from build123d import *

# Parameters (mm, degrees)
F0_W     = 10
F0_H     = 15
F1_DEPTH = 5
F2_DEPTH = 3
F4_DEPTH = 3
F5_DEPTH = 25


with BuildPart() as f1:
    # F0 (on Top) → F1 (new body)
    with BuildSketch(Plane.XY):
        Rectangle(F0_W, F0_H)
    extrude(amount=-F1_DEPTH)

    # F0 (on Top) → F2 (join)
    with BuildSketch(Plane.XY):
        with BuildLine():
            Line((-30, -50), (30, -50))
            Line((30, -50), (30, 50))
            Line((30, 50), (15, 50))
            Line((15, 50), (15, 46.55))
            ThreePointArc((15, 46.55), (16.0960155108, 46.0960155108), (16.55, 45))
            ThreePointArc((16.55, 45), (16.2263348543, 44.0520533638), (15.3905124838, 43.5))
            Line((15.3905124838, 43.5), (20.76, 43.5))
            Line((20.76, 43.5), (23.935, 43.5))
            Line((23.935, 43.5), (27.5, 43.5))
            Line((27.5, 43.5), (27.5, -43.5))
            Line((27.5, -43.5), (-27.5, -43.5))
            Line((-27.5, -43.5), (-27.5, -37.145))
            Line((-27.5, -37.145), (-27.5, 28.895))
            Line((-27.5, 28.895), (-27.5, 43.5))
            Line((-27.5, 43.5), (-24.325, 43.5))
            Line((-24.325, 43.5), (-21.15, 43.5))
            Line((-21.15, 43.5), (-15.3905124838, 43.5))
            ThreePointArc((-15.3905124838, 43.5), (-16.2263348543, 44.0520533638), (-16.55, 45))
            Line((-16.55, 45), (-30, 45))
            Line((-30, 45), (-30, -50))
        make_face()
        with BuildLine():
            Line((-30, 50), (-30, 45))
            Line((-30, 45), (-16.55, 45))
            ThreePointArc((-16.55, 45), (-16.0960155108, 46.0960155108), (-15, 46.55))
            Line((-15, 46.55), (-15, 50))
            Line((-15, 50), (-30, 50))
        make_face()
        with BuildLine():
            Line((15, 46.55), (15, 50))
            Line((15, 50), (-15, 50))
            Line((-15, 50), (-15, 46.55))
            ThreePointArc((-15, 46.55), (-13.9039844892, 46.0960155108), (-13.45, 45))
            Line((-13.45, 45), (13.45, 45))
            ThreePointArc((13.45, 45), (13.9039844892, 46.0960155108), (15, 46.55))
        make_face()
        with BuildLine():
            ThreePointArc((-14.6094875162, 43.5), (-15, 43.45), (-15.3905124838, 43.5))
            Line((-15.3905124838, 43.5), (-21.15, 43.5))
            Line((-21.15, 43.5), (-21.15, 28.895))
            Line((-21.15, 28.895), (20.76, 28.895))
            Line((20.76, 28.895), (20.76, 43.5))
            Line((20.76, 43.5), (15.3905124838, 43.5))
            ThreePointArc((15.3905124838, 43.5), (15, 43.45), (14.6094875162, 43.5))
            Line((14.6094875162, 43.5), (-14.6094875162, 43.5))
        make_face()
        with BuildLine():
            ThreePointArc((14.6094875162, 43.5), (13.7736651457, 44.0520533638), (13.45, 45))
            Line((13.45, 45), (-13.45, 45))
            ThreePointArc((-13.45, 45), (-13.7736651457, 44.0520533638), (-14.6094875162, 43.5))
            Line((-14.6094875162, 43.5), (14.6094875162, 43.5))
        make_face()
        with BuildLine():
            Line((-21.15, 28.895), (-21.15, 43.5))
            Line((-21.15, 43.5), (-24.325, 43.5))
            Line((-24.325, 43.5), (-24.325, 30.445))
            ThreePointArc((-24.325, 30.445), (-23.2289844892, 29.9910155108), (-22.775, 28.895))
            Line((-22.775, 28.895), (-21.15, 28.895))
        make_face()
        with BuildLine():
            Line((-24.325, 30.445), (-24.325, 43.5))
            Line((-24.325, 43.5), (-27.5, 43.5))
            Line((-27.5, 43.5), (-27.5, 28.895))
            Line((-27.5, 28.895), (-25.875, 28.895))
            ThreePointArc((-25.875, 28.895), (-25.4210155108, 29.9910155108), (-24.325, 30.445))
        make_face()
        with BuildLine():
            Line((-21.15, -35.595), (-21.15, 28.895))
            Line((-21.15, 28.895), (-22.775, 28.895))
            ThreePointArc((-22.775, 28.895), (-24.325, 27.345), (-25.875, 28.895))
            Line((-25.875, 28.895), (-27.5, 28.895))
            Line((-27.5, 28.895), (-27.5, -37.145))
            Line((-27.5, -37.145), (-22.7, -37.145))
            ThreePointArc((-22.7, -37.145), (-22.2460155108, -36.0489844892), (-21.15, -35.595))
        make_face()
        with BuildLine():
            Line((20.76, 28.895), (-21.15, 28.895))
            Line((-21.15, 28.895), (-21.15, -35.595))
            ThreePointArc((-21.15, -35.595), (-20.0539844892, -36.0489844892), (-19.6, -37.145))
            Line((-19.6, -37.145), (19.21, -37.145))
            ThreePointArc((19.21, -37.145), (19.6639844892, -36.0489844892), (20.76, -35.595))
            Line((20.76, -35.595), (20.76, 28.895))
        make_face()
        Rectangle(F0_W, F0_H, mode=Mode.SUBTRACT)
        with BuildLine():
            Line((23.935, 43.5), (20.76, 43.5))
            Line((20.76, 43.5), (20.76, 28.895))
            Line((20.76, 28.895), (22.385, 28.895))
            ThreePointArc((22.385, 28.895), (22.8389844892, 29.9910155108), (23.935, 30.445))
            Line((23.935, 30.445), (23.935, 43.5))
        make_face()
        with BuildLine():
            Line((22.385, 28.895), (20.76, 28.895))
            Line((20.76, 28.895), (20.76, -35.595))
            ThreePointArc((20.76, -35.595), (21.8560155108, -36.0489844892), (22.31, -37.145))
            ThreePointArc((22.31, -37.145), (20.76, -38.695), (19.21, -37.145))
            Line((19.21, -37.145), (-19.6, -37.145))
            ThreePointArc((-19.6, -37.145), (-21.15, -38.695), (-22.7, -37.145))
            Line((-22.7, -37.145), (-27.5, -37.145))
            Line((-27.5, -37.145), (-27.5, -43.5))
            Line((-27.5, -43.5), (27.5, -43.5))
            Line((27.5, -43.5), (27.5, 43.5))
            Line((27.5, 43.5), (23.935, 43.5))
            Line((23.935, 43.5), (23.935, 30.445))
            ThreePointArc((23.935, 30.445), (25.0310155108, 29.9910155108), (25.485, 28.895))
            ThreePointArc((25.485, 28.895), (23.935, 27.345), (22.385, 28.895))
        make_face()
        Rectangle(F0_W, F0_H)
    extrude(amount=F2_DEPTH)

    # F3 (on face) → F4 (join)
    with BuildSketch(Plane.XY.offset(3)):
        with BuildLine():
            Line((10, 50), (-10, 50))
            Line((-10, 50), (-10, 46.55))
            ThreePointArc((-10, 46.55), (-8.9039844892, 46.0960155108), (-8.45, 45))
            Line((-8.45, 45), (8.45, 45))
            ThreePointArc((8.45, 45), (8.9039844892, 46.0960155108), (10, 46.55))
            Line((10, 46.55), (10, 50))
        make_face()
        with BuildLine():
            Line((30, 50), (10, 50))
            Line((10, 50), (10, 46.55))
            ThreePointArc((10, 46.55), (11.0960155108, 46.0960155108), (11.55, 45))
            Line((11.55, 45), (13.45, 45))
            ThreePointArc((13.45, 45), (15, 46.55), (16.55, 45))
            Line((16.55, 45), (30, 45))
            Line((30, 45), (30, 50))
        make_face()
        with BuildLine():
            Line((-16.55, 45), (-30, 45))
            Line((-30, 45), (-30, 40))
            Line((-30, 40), (30, 40))
            Line((30, 40), (30, 45))
            Line((30, 45), (16.55, 45))
            ThreePointArc((16.55, 45), (15, 43.45), (13.45, 45))
            Line((13.45, 45), (11.55, 45))
            ThreePointArc((11.55, 45), (10, 43.45), (8.45, 45))
            Line((8.45, 45), (-8.45, 45))
            ThreePointArc((-8.45, 45), (-10, 43.45), (-11.55, 45))
            Line((-11.55, 45), (-13.45, 45))
            ThreePointArc((-13.45, 45), (-15, 43.45), (-16.55, 45))
        make_face()
        with BuildLine():
            Line((-13.45, 45), (-16.55, 45))
            ThreePointArc((-16.55, 45), (-15, 43.45), (-13.45, 45))
        make_face()
        with BuildLine():
            ThreePointArc((-13.45, 45), (-15, 46.55), (-16.55, 45))
            Line((-16.55, 45), (-13.45, 45))
        make_face()
        with BuildLine():
            Line((-10, 50), (-30, 50))
            Line((-30, 50), (-30, 45))
            Line((-30, 45), (-16.55, 45))
            ThreePointArc((-16.55, 45), (-15, 46.55), (-13.45, 45))
            Line((-13.45, 45), (-11.55, 45))
            ThreePointArc((-11.55, 45), (-11.0960155108, 46.0960155108), (-10, 46.55))
            Line((-10, 46.55), (-10, 50))
        make_face()
        with BuildLine():
            Line((13.45, 45), (16.55, 45))
            ThreePointArc((16.55, 45), (15, 46.55), (13.45, 45))
        make_face()
        with BuildLine():
            ThreePointArc((13.45, 45), (15, 43.45), (16.55, 45))
            Line((16.55, 45), (13.45, 45))
        make_face()
    extrude(amount=-F4_DEPTH)

    # F3 (on face) → F5 (cut)
    with BuildSketch(Plane.XY.offset(3)):
        with BuildLine():
            Line((-8.45, 45), (-10, 45))
            Line((-10, 45), (-11.55, 45))
            ThreePointArc((-11.55, 45), (-10, 43.45), (-8.45, 45))
        make_face()
        with BuildLine():
            ThreePointArc((-8.45, 45), (-8.9039844892, 46.0960155108), (-10, 46.55))
            Line((-10, 46.55), (-10, 45))
            Line((-10, 45), (-8.45, 45))
        make_face()
        with BuildLine():
            Line((-10, 45), (-10, 46.55))
            ThreePointArc((-10, 46.55), (-11.0960155108, 46.0960155108), (-11.55, 45))
            Line((-11.55, 45), (-10, 45))
        make_face()
        with BuildLine():
            ThreePointArc((11.55, 45), (11.0960155108, 46.0960155108), (10, 46.55))
            Line((10, 46.55), (10, 45))
            Line((10, 45), (11.55, 45))
        make_face()
        with BuildLine():
            Line((10, 45), (10, 46.55))
            ThreePointArc((10, 46.55), (8.9039844892, 46.0960155108), (8.45, 45))
            Line((8.45, 45), (10, 45))
        make_face()
        with BuildLine():
            Line((11.55, 45), (10, 45))
            Line((10, 45), (8.45, 45))
            ThreePointArc((8.45, 45), (10, 43.45), (11.55, 45))
        make_face()
    extrude(amount=-F5_DEPTH, mode=Mode.SUBTRACT)


solid = f1.part
Source: CAD feature listing. Evaluate the final solid. Frame: model axes, mm. A direction names the side the tool comes from. Round coordinates to 2 decimals unless told otherwise and drop trailing zeros. Loops run counter-clockwise (first coordinate to the right, second up) from the corner with the lowest first, then second, coordinate; pieces in that order, holes last. Notation, with made-up numbers: (29.25, 31.25) - (53.25, 31.25) arc R16 ccw to (53.25, 36.25) - close; hole circle Ø2 at (43, 89.5). An arc over 180 degrees is marked (long way). Write item = value, one per line. Start each with the question number.
Item 1: Section query B-B on y = 6. Output: boundary loops of the cut face in (x, z).
Item 2: First-contact query: pin 1 Ø12 at (x, y) = (10, -15) entering from -Z; pin 2 Ø2 at (y, z) = (3.5, -3) entering from -X; pin 3 Ø1.5 at (x, z) = (2, -3) entering from +Y. Flat tips, straight axial feed; report the tip coordinate or a pass-through.
Item 3: Section query A-A on x = -1. Output: boundary loops of the cut face in (y, z), plus the area to 3 significant figures.
Item 4: Material intervals for line 1 (X direction, y = 5.5, z = -3.5); line 2 (Z direction, x = 2.5, y = 37.5); line 3 (Y direction, x = -9.5, z = 0.25), sorted ascending.
Item 5: Section query D-D on y = -13. Output: boundary loops of the cut face in (x, z).
Item 6: Reachability of faces 1 (the face through (-5, 0, -2)), 2 (the face through (0, -7.5, -2)), 3 (the face through (0, 7.5, -2)), 4 (the face through (5, 0, -2)) from +Z, -Z, +X, -X, +Y, -Y: full face, straight path, thin tool, end or side. Return the list, or none.
Item 7: Section query C-C on z = -2.75. Output: boundary loops of the cut face in (x, y).
Results list:
q1.outline = (-30, 0) - (-5, 0) - (-5, -5) - (5, -5) - (5, 0) - (30, 0) - (30, 3) - (-30, 3) - close
q2.pin_1 = 0
q2.pin_2 = -5
q2.pin_3 = 7.5
q3.outline = (-50, 0) - (-7.5, 0) - (-7.5, -5) - (7.5, -5) - (7.5, 0) - (50, 0) - (50, 3) - (-50, 3) - close
q3.area = 375 mm²
q4.line_1 = -5 to 5
q4.line_2 = 0 to 3
q4.line_3 = -50 to 43.53, 46.47 to 50
q5.outline = (-30, 0) - (30, 0) - (30, 3) - (-30, 3) - close
q6.face_1 = -Z, -X, +Y, -Y
q6.face_2 = -Z, +X, -X, -Y
q6.face_3 = -Z, +X, -X, +Y
q6.face_4 = -Z, +X, +Y, -Y
q7.outline = (-5, -7.5) - (5, -7.5) - (5, 7.5) - (-5, 7.5) - close
